Autodesk Inventor part; units mm, degrees
ref_plane "YZ Plane" through (0, 0, 0) normal (1, 0, 0) x (0, 1, 0)
ref_plane "XZ Plane" through (0, 0, 0) normal (0, 1, 0) x (-1, 0, 0)
ref_plane "XY Plane" through (0, 0, 0) normal (0, 0, 1) x (1, 0, 0)
sketch "Sketch1" plane through (0, 0, 0) normal (0, 1, 0) x (-1, 0, 0)
  circle A0 centre (0, 0) radius 10
  dimension "d0" = 20
extrude "Extrusion1" add sketch "Sketch1" along normal blind 15
sketch "Sketch2" plane through (0, 15, 0) normal (0, 1, 0) x (1, 0, 0)
  circle A0 centre (0, 0) radius 8.5
  dimension "d5" = 17
extrude "Extrusion2" cut sketch "Sketch2" against normal blind 1
sketch "Sketch3" plane through (0, 14, 0) normal (0, 1, 0) x (1, 0, 0)
  circle A0 centre (0, 0) radius 4
  dimension "d8" = 8
extrude "Extrusion3" add sketch "Sketch3" along normal blind 1
sketch "Sketch4" plane through (0, 0, 0) normal (0, -1, 0) x (1, 0, 0)
  circle A0 centre (0, 0) radius 2
  dimension "d11" = 4
extrude "Extrusion4" cut sketch "Sketch4" against normal blind 5
sketch "Sketch5" plane through (0, 0, 0) normal (0, -1, 0) x (1, 0, 0)
  point P0 (0, 0)
fillet "Fillet1" radius 1 1 edges at (-2, 0, 0)
thread "Thread1"
properties part number "Eletroima" material "Iron, Cast"
Part model, mm, in its own coordinate system. A direction names the side the tool comes from. Round coordinates to 2 decimals unless told otherwise and drop trailing zeros. Order: outer loops, then holes, each group sorted by start corner. A loop starts at its lowest first (then second) coordinate and runs counter-clockwise, first axis right, second up. Notation, with made-up numbers: M 25,62 L 40,62 A12 cw 40,75 Z; hole C 37,82.25 d7. An arc over 180 degrees is marked long. Put each result on its own line as item: value. Start each with the question number.
1. Slice it at B-B on x = 0. List the corners of the cut face in (y, z), then the cut area to 3 significant figures.
2. Two-plate mould, pull along X, no slides. Class faces 1 (the face through (-0.867, 14.493, -3.905)), 2 (the face through (2.17, 7.4, 9.76)), 3 (the face through (-2.1, 0, 2.4)), 4 (the face through (0, 3, -2)): +X half, -X half, draft (parallel to the pull), parting line (faces both ways), or undercut.
3. Tool access for faces 5 (the face through (0, 15, 0)), 6 (the face through (4.57, 14.507, -7.167)), 7 (the face through (0, 5, 0)): list every direction of +Z, -Z, +X, -X, +Y, -Y with a clear straight run to the whole face (end or side of a thin tool).
4. Slice it at A-A on y = 3. List the corners of the cut face in (x, z), then the cut area to 3 significant figures.
5. Slice it at C-C on z = 0. List the corners of the cut face in (x, y).
6. Drill centre lines: probe 1 along Z at (x, y) = (0, 14.7); probe 2 along Z at (x, y) = (0, 3.1); probe 3 along Y at (x, z) = (2.5, -6.25). Where is each one in solid material? Low to high. Write a range as [from, to].
7. Drop flat-ended pins along their axis: pin 1 (2 mm diameter, centred on x = -8, y = 2, fed in from +Z); pin 2 (4.5 mm diameter, centred on x = 0.5, z = 0, fed in from -Y); pin 3 (1 mm diameter, centred on x = -3, z = -5.5, fed in from +Y). Give the stop position or say it passes through.
8. Slice it at D-D on y = 5.5. List the corners of the cut face in (x, z).
Findings:
1. outline: M 0,-10 L 15,-10 L 15,-8.5 L 14,-8.5 L 14,-4 L 15,-4 L 15,4 L 14,4 L 14,8.5 L 15,8.5 L 15,10 L 0,10 L 0,3 A1 ccw 1,2 L 5,2 L 5,-2 L 1,-2 A1 ccw 0,-3 Z
1. area: 271 mm2
2. face 1: undercut
2. face 2: parting line
2. face 3: draft
2. face 4: undercut
3. face 5: +Z, -Z, +X, -X, +Y
3. face 6: +Y
3. face 7: -Y
4. outline: C 0,0 d20; hole C 0,0 d4
4. area: 302 mm2
5. outline: M -10,0 L -3,0 A1 ccw -2,1 L -2,5 L 2,5 L 2,1 A1 ccw 3,0 L 10,0 L 10,15 L 8.5,15 L 8.5,14 L 4,14 L 4,15 L -4,15 L -4,14 L -8.5,14 L -8.5,15 L -10,15 Z
6. probe 1: [-10, -8.5], [-4, 4], [8.5, 10]
6. probe 2: [-10, -2], [2, 10]
6. probe 3: [0, 14]
7. pin 1: z = 7.14
7. pin 2: y = 0.03
7. pin 3: y = 14
8. outline: C 0,0 d20
